Geometry check sheet. Reference: the model listing, model coordinates, mm. Face numbers are marked on the shaded views. A direction names the side the tool comes from. Round coordinates to 2 decimals unless told otherwise and drop trailing zeros. Order: outer loops, then holes, each group sorted by start corner. A loop starts at its lowest first (then second) coordinate and runs counter-clockwise, first axis right, second up. Notation, with made-up numbers: (-14, 53.25) - (4, 53.25) arc R21 ccw to (4, 68.25) - close; hole circle Ø3 at (14.25, 73). An arc over 180 degrees is marked (long way). One line per question, with ' | ' between items. Start each with the question number.
Q1. Sectioned sample at A-A, the plane z = -3.5. Enter the section's corners in (x, y), then the cut area to 3 significant figures.
Q2. Material ranges on line 1 along X through (y, z) = (-34.25, -6); line 2 along Y through (x, z) = (-3.1, -5.25); line 3 along Z through (x, y) = (-0.85, -34.75), recorded low to high.
Q3. Sectioned sample at B-B, the plane y = -31.5. Enter the section's corners in (x, z), then the cut area to 3 significant figures.
Q4. Tool access check on the marked faces 1, 2, 3, 4 and 5. Record the directions out of +Z, -Z, +X, -X, +Y, -Y that give a thin tool (end or side, any length) a straight path to the whole face; none if there is none.
Q5. Sectioned sample at C-C, the plane z = -1. Enter the section's corners in (x, y).
Q6. Mould release check, pull along X, two halves, no side actions. Record for the marked faces 6, 7 and 8: +X half, -X half, draft (parallel to the pull), parting line (faces both ways), or undercut.
Q7. Gauge pin test, flat ends, axial feed: P1, Ø1.5, axis at y = -34, z = -1, coming from the -X side; P2, Ø2.5, axis at y = -35, z = -5.5, coming from the -X side; P3, Ø2.5, axis at y = -35.5, z = -5, coming from the +X side. Record the tip position at first contact, or that the pin passes through.
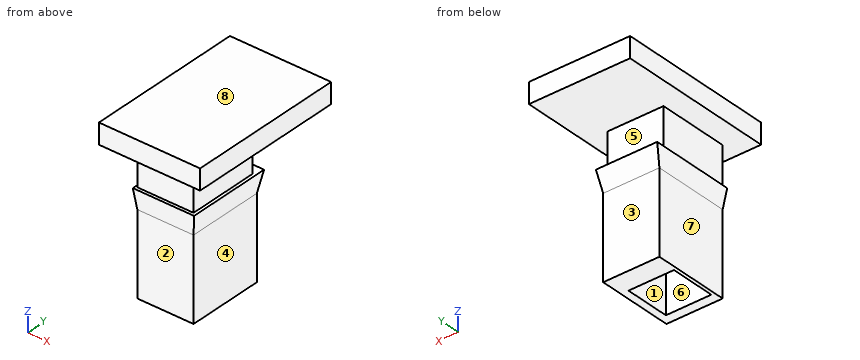
```python
from build123d import *

# Parameters (mm, degrees)
EXTRUDE_1_DEPTH      = 0.2
EXTRUDE_1_DEPTH_BACK = 1.7
SKETCH_2_W           = 2.749
SKETCH_2_H           = 3.486646178
SKETCH_3_W           = 4.948986656
SKETCH_3_H           = 7.726872963
EXTRUDE_2_DEPTH      = 1
SKETCH_8_W           = 2.749
SKETCH_8_H           = 3.729608675
EXTRUDE_3_DEPTH      = 4
SKETCH_9_W           = 2.220876602
SKETCH_9_H           = 2.202369297
CUT_EXTRUDE_1_DEPTH  = 3.5


with BuildPart() as part:
    # 草图2 → 凸台-拉伸1 (new, two sides: drawn at the far end of the back side and taken through both)
    with BuildSketch(Plane.XY.offset(-EXTRUDE_1_DEPTH_BACK)):
        with Locations((-2.824500159, -34.686907223)):
            Rectangle(SKETCH_2_W, SKETCH_2_H)
    extrude(amount=EXTRUDE_1_DEPTH + EXTRUDE_1_DEPTH_BACK)

    # 草图3 → 凸台-拉伸2 (add)
    with BuildSketch(Plane.XY.offset(0.2)):
        with Locations((-2.854795759, -33.471663218)):
            Rectangle(SKETCH_3_W, SKETCH_3_H)
    extrude(amount=EXTRUDE_2_DEPTH)

    # 放样1: read off the stored shape, not the designer's step
    # 放样1: loft between two sections, ruled curve by curve
    loft_1_from = [
        Edge.make_line((-1.450000159, -32.700621637, -2.7), (-1.450000159, -36.430230312, -2.7)),
        Edge.make_line((-1.450000159, -36.430230312, -2.7), (-4.199000159, -36.430230312, -2.7)),
        Edge.make_line((-4.199000159, -36.430230312, -2.7), (-4.199000159, -32.700621637, -2.7)),
        Edge.make_line((-4.199000159, -32.700621637, -2.7), (-1.450000159, -32.700621637, -2.7)),
    ]
    loft_1_to = [
        Edge.make_line((-1.300000159, -32.449611662, -1.7), (-1.300000159, -36.579532352, -1.7)),
        Edge.make_line((-1.300000159, -36.579532352, -1.7), (-4.299000159, -36.579532352, -1.7)),
        Edge.make_line((-4.299000159, -36.579532352, -1.7), (-4.299000159, -32.449611662, -1.7)),
        Edge.make_line((-4.299000159, -32.449611662, -1.7), (-1.300000159, -32.449611662, -1.7)),
    ]
    loft_1 = Solid(Shell([*[Face.make_surface_from_curves(loft_1_from[k], loft_1_to[k]) for k in range(4)], Face(Wire(loft_1_from)), Face(Wire(loft_1_to))]))
    add(loft_1)

    # 草图8 → 凸台-拉伸3 (add)
    with BuildSketch(Plane(origin=(0, 0, -2.7), x_dir=(-1, 0, 0), z_dir=(0, 0, -1))):
        with Locations((2.824500159, -34.565425975)):
            Rectangle(SKETCH_8_W, SKETCH_8_H)
    extrude(amount=EXTRUDE_3_DEPTH)

    # 草图9 → 切除-拉伸1 (cut)
    with BuildSketch(Plane(origin=(0, 0, -6.7), x_dir=(-1, 0, 0), z_dir=(0, 0, -1))):
        with Locations((2.92610545, -34.854711182)):
            Rectangle(SKETCH_9_W, SKETCH_9_H)
    extrude(amount=-CUT_EXTRUDE_1_DEPTH, mode=Mode.SUBTRACT)


solid = part.part
```
Determined:
1) outline: (-4.2, -36.43) - (-1.45, -36.43) - (-1.45, -32.7) - (-4.2, -32.7) - close; hole (-4.04, -35.96) - (-1.82, -35.96) - (-1.82, -33.75) - (-4.04, -33.75) - close | area: 5.36 mm2
2) line 1: x = -4.2 to -4.04, -1.82 to -1.45 | line 2: y = -36.43 to -35.96, -33.75 to -32.7 | line 3: z = 0.2 to 1.2
3) outline: (-5.33, 0.2) - (-0.38, 0.2) - (-0.38, 1.2) - (-5.33, 1.2) - close | area: 4.95 mm2
4) face 1: -Z | face 2: -Z, +X, -X, -Y | face 3: -Z, +X, -X, +Y | face 4: -Z, +X, +Y, -Y | face 5: +X, -X, +Y
5) outline: (-4.2, -36.43) - (-1.45, -36.43) - (-1.45, -32.94) - (-4.2, -32.94) - close
6) face 6: undercut | face 7: -X half | face 8: draft
7) P1: stops at x = -4.3 | P2: stops at x = -4.2 | P3: stops at x = -1.45
